Model file for the job. Use its own axes, mm. A direction names the side the tool comes from. Coordinates: 2 decimals unless noted, no trailing zeros. Write each loop counter-clockwise with the first axis right and the second up, starting at its lowest first coordinate (ties: lowest second). Pieces come first, ordered by that corner, then holes. Notation, with made-up numbers: (45, 46) - (102, 46) arc R33 ccw to (102, 83) - close; hole circle Ø7 at (49, 6). An arc over 180 degrees is marked (long way). Put each result on its own line as item: value. Start each with the question number.
1. Drill centre lines: L1, parallel to X at y = -44, z = -38.5; L2, parallel to X at y = -64, z = -11.5; L3, parallel to X at y = -165, z = -26. Where is each one in solid material? Low to high. Write a range as from..to.
2. Pull direction X, two halves, no side cores. Call faces 1 (the face through (98.286, -94, -55)), 2 (the face through (415.762, -92, -13)), 3 (the face through (30, -181.61, -29)): released by +X, released by -X, zero draft, split by the parting line, or undercut.
3. Saw through at A-A, the plane y = -76. Write the cut outline in (x, z).
4. Saw through at C-C, the plane x = -8. Write the cut outline in (y, z).
5. Which spindle directions (+Z, -Z, +X, -X, +Y, -Y) get a long thin tool onto all of the face, cutting with end or side? Do faces 4 (the face through (263, -92, 64.649)), 5 (the face through (79, -3.556, -55)), 6 (the face through (-21.52, -89.53, 31.53)), 7 (the face through (-3, -92, -22.049)), 8 (the face through (77, -3.556, 76)). Say none if no direction does.
6. Saw through at B-B, the plane z = -56. Write the cut outline in (x, y).
7. Drop flat-ended pins along their axis: P1, Ø10, axis at x = 277, y = -89.5, coming from the +Z side; P2, Ø21.5, axis at x = 86.5, z = 81, coming from the +Y side; P3, Ø3, axis at x = -62, y = -70.5, coming from the +Z side. Give the stop position or say it passes through.
8. Saw through at D-D, the plane z = 30. Write the cut outline in (x, y), plus the area to 3 significant figures.
```python
from build123d import *

# Parameters (mm, degrees)
F1_DEPTH  = 25.4
F2_DEPTH  = 105.41
F4_DEPTH  = 25.4
F7_DEPTH  = 34.544
F8_DEPTH  = 25.4
F9_W      = 33.2944607362
F9_H      = 55.5258449167
F10_DEPTH = 25.4
F11_DEPTH = 249.682
F12_W     = 53.8298841566
F12_H     = 169.9287788942
F12_W_2   = 19.2790124565
F13_DEPTH = 1.524
F14_DEPTH = 70.866
F16_W     = 37.628442049
F16_H     = 45.0919307768
F17_DEPTH = 178.054
F18_DEPTH = 53.594
F20_DEPTH = 178.054
F22_DEPTH = 181.102
F23_DEPTH = 302.26
F24_DEPTH = 302.26
F25_DEPTH = 142.24
F26_DEPTH = 142.24


with BuildPart() as f1:
    # F0 (on Front) → F1 (new body)
    with BuildSketch(Plane.XZ):
        Polygon((-43.6498820782, -77.5746703148), (42.2929041088, -77.5746703148), (42.2929041088, 0), (0, 62.1954351664), (-43.6498820782, 0), align=None)
    extrude(amount=F1_DEPTH)

    # F2 (add): a face of the model
    f2_faces = [f1.faces().sort_by_distance(p)[0] for p in [
        (-0.6137701258, -25.4, -21.7553212645),
    ]]
    extrude(f2_faces, amount=F2_DEPTH)

    # F3 (on face) → F4 (join)
    with BuildSketch(Plane.XZ.offset(130.81)):
        Polygon((-43.6498820782, 0), (-43.6498820782, -77.5746703148), (42.2929041088, -77.5746703148), (42.2929041088, 0), (0, 62.1954351664), align=None)
    extrude(amount=F4_DEPTH)

    # F6 (on face) → F7 (join)
    with BuildSketch(Plane.XZ.offset(156.21)):
        Polygon((-16.9418714941, -35.6023237109), (-16.9418714941, -77.5746703148), (13.7008177117, -77.5746703148), (13.7008177117, -37.0755307376), (13.7008177117, -35.6023237109), align=None)
    extrude(amount=-F7_DEPTH)

    # F5 (on face) → F8 (join)
    with BuildSketch(Plane.XZ.offset(156.21)):
        Polygon((-17.8257934749, -77.5746703148), (13.7008177117, -77.5746703148), (42.2929041088, -77.5746703148), (42.2929041088, 0), (0, 62.1954351664), (-43.6498820782, 0), (-43.6498820782, -77.5746703148), align=None)
    extrude(amount=F8_DEPTH)

    # F9 (on face) → F10 (join)
    with BuildSketch(Plane.XZ.offset(181.61)):
        with Locations((-2.3571313359, -49.8117478564)):
            Rectangle(F9_W, F9_H)
    extrude(amount=F10_DEPTH)

    # F11 (cut): a face of the model
    f11_faces = [f1.faces().sort_by_distance(p)[0] for p in [
        (-2.3571313359, -207.01, -49.8117478564),
    ]]
    extrude(f11_faces, amount=-F11_DEPTH, mode=Mode.SUBTRACT)

    # F12 (on face) → F13 (join)
    with BuildSketch(Plane(origin=(0, 0, -77.5746703148), x_dir=(1, 0, 0), z_dir=(0, 0, -1))):
        with Locations((7.9105803743, 90.9883729182)):
            Rectangle(F12_W, F12_H)
        with Locations((-28.6438679323, 90.9883729182)):
            Rectangle(F12_W_2, F12_H)
    extrude(amount=-F13_DEPTH)

    # F14 (add): a face of the model
    f14_faces = [f1.faces().sort_by_distance(p)[0] for p in [
        (42.2929041088, -90.805, -38.7873351574),
    ]]
    extrude(f14_faces, amount=F14_DEPTH)

    # F16 (on face) → F17 (cut)
    with BuildSketch(Plane.XZ.offset(181.61)):
        with Locations((79.4716104865, -54.9975987524)):
            Rectangle(F16_W, F16_H)
    extrude(amount=-F17_DEPTH, mode=Mode.SUBTRACT)

    # F18 (add): a face of the model
    f18_faces = [f1.faces().sort_by_distance(p)[0] for p in [
        (77.7259041088, -90.805, 0),
    ]]
    extrude(f18_faces, amount=F18_DEPTH)

    # F19 (on face) → F20 (join)
    with BuildSketch(Plane.XZ.offset(181.61)):
        Polygon((79.4050395489, 130.5681169033), (42.2929041088, 53.594), (113.1589041088, 53.594), align=None)
    extrude(amount=-F20_DEPTH)

    # F21 (on face) → F22 (join)
    with BuildSketch(Plane.XZ.offset(181.61)):
        Polygon((-43.6498820782, -76.761349558), (-43.8248664141, -76.7604261637), (-43.8248664141, -87.9684388638), (113.5024726391, -87.9684388638), (113.5024726391, -77.5906443596), (42.2929041088, -77.2148706392), (42.2929041088, -77.5746703148), (14.2900990322, -77.5746703148), (14.2900990322, -77.0670995115), (-19.004361704, -76.8914042554), (-19.004361704, -77.5746703148), (-43.6498820782, -77.5746703148), align=None)
    extrude(amount=-F22_DEPTH)

    # F23 (add): a face of the model
    f23_faces = [f1.faces().sort_by_distance(p)[0] for p in [
        (-43.8248664141, -91.059, -82.3644325137),
    ]]
    extrude(f23_faces, amount=F23_DEPTH)

    # F24 (add): a face of the model
    f24_faces = [f1.faces().sort_by_distance(p)[0] for p in [
        (113.5024726391, -91.059, -82.7795416117),
    ]]
    extrude(f24_faces, amount=F24_DEPTH)

    # F25 (add): a face of the model
    f25_faces = [f1.faces().sort_by_distance(p)[0] for p in [
        (-194.9548664141, -91.059, -76.7604261637),
    ]]
    extrude(f25_faces, amount=F25_DEPTH)

    # F26 (add): a face of the model
    f26_faces = [f1.faces().sort_by_distance(p)[0] for p in [
        (264.6324726391, -91.059, -77.5906443596),
    ]]
    extrude(f26_faces, amount=F26_DEPTH)


solid = f1.part
```
Final values:
1. L1: x = -346.08..-43.82, -43.65..-19, 14.29..60.66, 98.29..113.16, 113.5..415.76
1. L2: x = -346.08..-43.82, -43.65..113.16, 113.5..415.76
1. L3: x = -346.08..-43.82, -43.65..-19, 14.29..113.16, 113.5..415.76
2. face 1: undercut
2. face 2: released by +X
2. face 3: zero draft
3. outline: (-346.08, -87.97) - (415.76, -87.97) - (415.76, 64.65) - (113.5, 64.65) - (113.5, -77.59) - (110.48, -77.57) - (113.16, -77.57) - (113.16, 53.59) - (79.41, 130.57) - (42.29, 53.59) - (42.29, 0) - (0, 62.2) - (-43.65, 0) - (-43.65, -76.76) - (-43.82, -76.76) - (-43.82, 65.48) - (-346.08, 65.48) - close; hole (-19, -76.05) - (14.29, -76.05) - (14.29, -22.05) - (-19, -22.05) - close; hole (60.66, -77.31) - (98.29, -77.51) - (98.29, -32.45) - (60.66, -32.45) - close
4. outline: (-181.61, -87.97) - (-0.51, -87.97) - (-0.51, -76.95) - (-6.02, -76.95) - (-6.02, -76.05) - (-175.95, -76.05) - (-175.95, -76.95) - (-181.61, -76.95) - close; (-181.61, -22.05) - (0, -22.05) - (0, 50.8) - (-181.61, 50.8) - close
5. face 4: +Z, +X, +Y, -Y
5. face 5: -Y
5. face 6: +Z, +Y, -Y
5. face 7: +Y, -Y
5. face 8: +Z, +Y
6. outline: (-346.08, -181.61) - (-43.82, -181.61) - (-43.82, -0.51) - (-346.08, -0.51) - close; (-43.65, -181.61) - (-19, -181.61) - (-19, 0) - (-43.65, 0) - close; (14.29, -181.61) - (60.66, -181.61) - (60.66, -3.56) - (98.29, -3.56) - (98.29, -181.61) - (113.16, -181.61) - (113.16, 0) - (14.29, 0) - close; (113.5, -181.61) - (415.76, -181.61) - (415.76, -0.51) - (113.5, -0.51) - close
7. P1: stops at z = 64.65
7. P2: stops at y = -3.56
7. P3: stops at z = 65.48
8. outline: (-346.08, -181.61) - (-43.82, -181.61) - (-43.82, -0.51) - (-346.08, -0.51) - close; (-22.6, -181.61) - (21.89, -181.61) - (21.89, 0) - (-22.6, 0) - close; (42.29, -181.61) - (113.16, -181.61) - (113.16, 0) - (42.29, 0) - close; (113.5, -181.61) - (415.76, -181.61) - (415.76, -0.51) - (113.5, -0.51) - close
8. area: 130,000 mm²
